Can you work these out from the drawing? Everything is in mm from the part's minimum corner. Round coordinates to 2 decimals unless told otherwise and drop trailing zeros. Loops run counter-clockwise (first coordinate to the right, second up) from the corner with the lowest first, then second, coordinate; pieces in that order, holes last. Notation, with made-up numbers: (14.5, 78) -> (36.5, 78) arc R31 ccw to (36.5, 106) -> close; hole circle Ø2 at (-17.75, 26). An arc over 180 degrees is marked (long way). Answer as a JSON object with one key per item and string values.
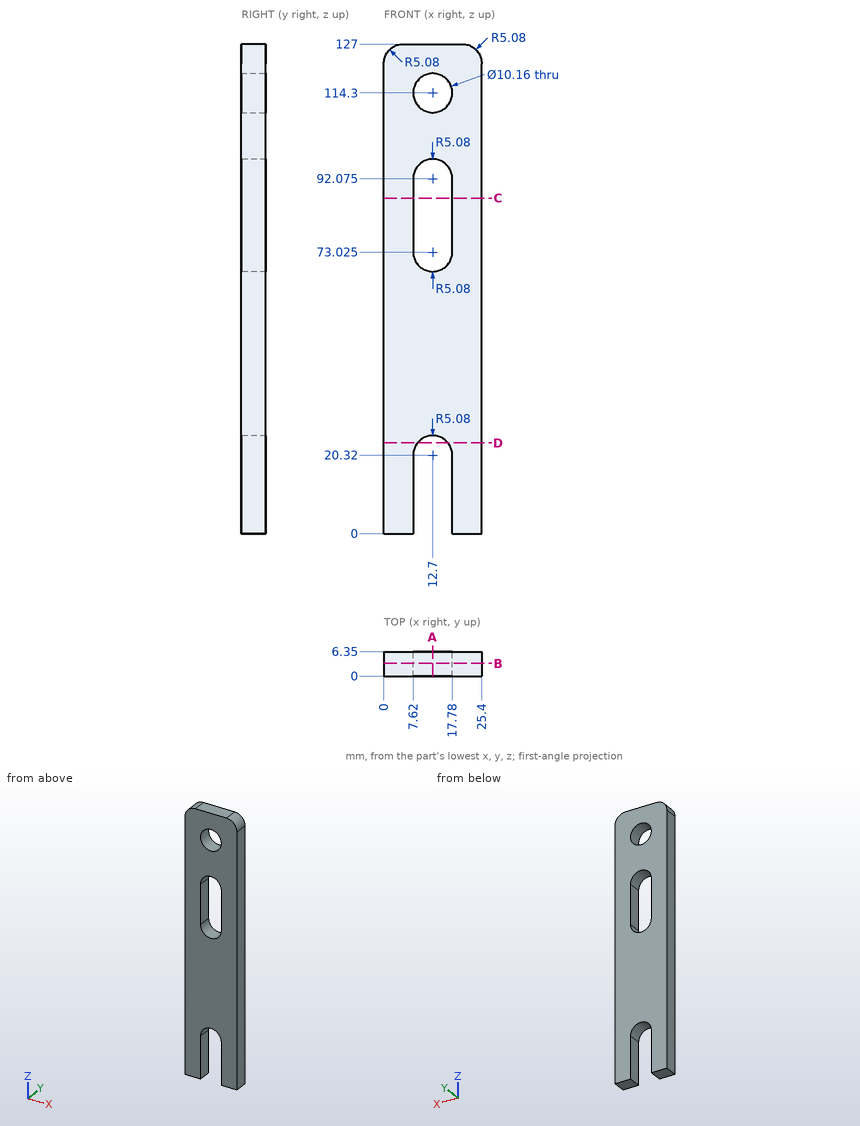
Q1. I'm going to push a flat-ended pin straight in: pin 1 (6 mm diameter, centred on x = 12.7, z = 114.3, fed in from +Y). Where does the tip first touch, or does it pass through?
Determined:
{"pin 1": "through"}
Q2. I want a section at B-B, the plane y = 3.25. Write out the boundary of the cut face in (x, z) (3 decimals).
Determined:
{"outline": "(0, 0) -> (7.62, 0) -> (7.62, 20.32) arc R5.08 cw to (17.78, 20.32) -> (17.78, 0) -> (25.4, 0) -> (25.4, 121.92) arc R5.08 ccw to (20.32, 127) -> (5.08, 127) arc R5.08 ccw to (0, 121.92) -> close; hole (7.62, 73.025) arc R5.08 ccw to (17.78, 73.025) -> (17.78, 92.075) arc R5.08 ccw to (7.62, 92.075) -> close; hole circle Ø10.16 at (12.7, 114.3)"}
Q3. If I drill on L1, parallel to Z at x = 12.75, y = 0.75; L2, parallel to Z at x = 13, y = 6.25; L3, parallel to X at y = 3.75, z = 12, over which ranges is the centre line in solid material (lowest first)? Write a range as [from, to].
Determined:
{"L1": "[25.4, 67.95], [97.15, 109.22], [119.38, 127]", "L2": "[25.39, 67.95], [97.15, 109.23], [119.37, 127]", "L3": "[0, 7.62], [17.78, 25.4]"}
Q4. I want a section at C-C, the plane z = 87. Write out the boundary of the cut face in (x, y), then the cut area to 3 significant figures.
Determined:
{"outline": "(0, 0) -> (7.62, 0) -> (7.62, 6.35) -> (0, 6.35) -> close; (17.78, 0) -> (25.4, 0) -> (25.4, 6.35) -> (17.78, 6.35) -> close", "area": "96.8 mm²"}
Q5. I want a section at A-A, the plane x = 12.7. Write out the boundary of the cut face in (y, z) (3 decimals), then the cut area to 3 significant figures.
Determined:
{"outline": "(0, 25.4) -> (6.35, 25.4) -> (6.35, 67.945) -> (0, 67.945) -> close; (0, 97.155) -> (6.35, 97.155) -> (6.35, 109.22) -> (0, 109.22) -> close; (0, 119.38) -> (6.35, 119.38) -> (6.35, 127) -> (0, 127) -> close", "area": "395 mm²"}
Q6. I want a section at D-D, the plane z = 23.5. Write out the boundary of the cut face in (x, y), then the cut area to 3 significant figures.
Determined:
{"outline": "(0, 0) -> (8.74, 0) -> (8.74, 6.35) -> (0, 6.35) -> close; (16.66, 0) -> (25.4, 0) -> (25.4, 6.35) -> (16.66, 6.35) -> close", "area": "111 mm²"}
